For this review, take the finished solid that the model builds, in its own axes (mm). Face numbers are marked on the shaded views. Coordinates: 2 decimals unless noted, no trailing zeros. Write each loop counter-clockwise with the first axis right and the second up, starting at its lowest first coordinate (ties: lowest second). Pieces come first, ordered by that corner, then holes.
1) We need section A-A on x = 0. Write out the cut boundary in (y, z).
2) We need section C-C on y = 2.3. Write out the cut boundary in (x, z), then the cut area to 3 significant figures.
3) We need section D-D on y = 0.7. Write out the cut boundary in (x, z).
4) Insertion check: P1, Ø1.6, axis at y = 1.5, z = 3, coming from the -X side; P2, Ø1.5, axis at x = 7, z = -4.5, coming from the -Y side; P3, Ø1, axis at y = 2, z = -0.5, coming from the +X side. Each pin has a flat end and moves straight along its axis. Give the tip position at first contact, or say it passes through.
5) To check wall thickness, follow line 1 along X through (y, z) = (1.05, 0.25); line 2 along X through (y, z) = (1.8, -2.5); line 3 along Z through (x, y) = (-6, 1.55). State the ranges of each line that lie inside material, in increasing order.
6) We need section B-B on z = 0. Write out the cut boundary in (x, y).
7) Mouldability with a two-part tool opening along X and no side actions: class the marked faces 1 and 2 as pulls with the +X half, pulls with the -X half, needs draft (parallel to the pull), parting line crosses it, or undercut.
from build123d import *

# Parameters (mm, degrees)
SKETCH1_R             = 13
SKETCH1_W             = 15.2
SKETCH1_H             = 13
BOSS_EXTRUDE1_DEPTH   = 3
FILLET1_R             = 2
CHAMFER1_SIZE         = 1
CHAMFER1_SIZE2        = 0.577350269
CHAMFER1_PART_2_SIZE  = 1
CHAMFER1_PART_2_SIZE2 = 0.577350269
CHAMFER1_PART_3_SIZE  = 1
CHAMFER1_PART_3_SIZE2 = 0.577350269
CHAMFER1_PART_4_SIZE  = 1
CHAMFER1_PART_4_SIZE2 = 0.577350269


with BuildPart() as part:
    # Sketch1 → Boss-Extrude1 (new body)
    with BuildSketch(Plane(origin=(0, 0, 0), x_dir=(1, 0, 0), z_dir=(0, 1, 0))):
        Circle(SKETCH1_R)
        Rectangle(SKETCH1_W, SKETCH1_H, mode=Mode.SUBTRACT)
    extrude(amount=BOSS_EXTRUDE1_DEPTH)

    # Fillet1
    fillet1_edges = [part.edges().sort_by_distance(p)[0] for p in [
        (-13, 3, 0),
    ]]
    fillet(fillet1_edges, radius=FILLET1_R)

    # Chamfer1
    chamfer1_edges = [part.edges().sort_by_distance(p)[0] for p in [
        (-7.6, 0, 0),
    ]]
    chamfer1_side = [part.faces().sort_by_distance(p)[0] for p in [
        (-7.6, 1.5, 0),
    ]]
    chamfer(chamfer1_edges, length=CHAMFER1_SIZE, length2=CHAMFER1_SIZE2, reference=chamfer1_side[0])

    # Chamfer1 part 2
    chamfer1_part_2_edges = [part.edges().sort_by_distance(p)[0] for p in [
        (0, 0, 6.5),
    ]]
    chamfer1_part_2_side = [part.faces().sort_by_distance(p)[0] for p in [
        (0, 1.5, 6.5),
    ]]
    chamfer(chamfer1_part_2_edges, length=CHAMFER1_PART_2_SIZE, length2=CHAMFER1_PART_2_SIZE2, reference=chamfer1_part_2_side[0])

    # Chamfer1 part 3
    chamfer1_part_3_edges = [part.edges().sort_by_distance(p)[0] for p in [
        (7.6, 0, 0),
    ]]
    chamfer1_part_3_side = [part.faces().sort_by_distance(p)[0] for p in [
        (7.6, 1.5, 0),
    ]]
    chamfer(chamfer1_part_3_edges, length=CHAMFER1_PART_3_SIZE, length2=CHAMFER1_PART_3_SIZE2, reference=chamfer1_part_3_side[0])

    # Chamfer1 part 4
    chamfer1_part_4_edges = [part.edges().sort_by_distance(p)[0] for p in [
        (0, 0, -6.5),
    ]]
    chamfer1_part_4_side = [part.faces().sort_by_distance(p)[0] for p in [
        (0, 1.5, -6.5),
    ]]
    chamfer(chamfer1_part_4_edges, length=CHAMFER1_PART_4_SIZE, length2=CHAMFER1_PART_4_SIZE2, reference=chamfer1_part_4_side[0])


solid = part.part
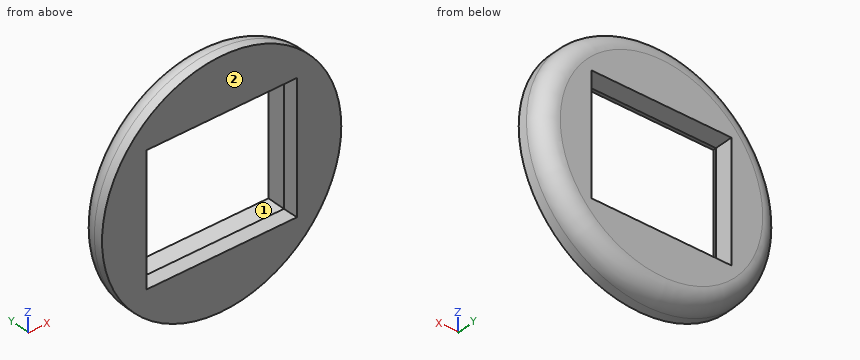
Result:
1. outline: (0, -13) - (1, -13) arc R2 ccw to (3, -11) - (3, -6.5) - (1, -6.5) - (0, -7.08) - close; (0, 7.08) - (1, 6.5) - (3, 6.5) - (3, 11) arc R2 ccw to (1, 13) - (0, 13) - close
2. outline: circle Ø25.04 at (0, 0); hole (-7.6, -6.5) - (7.6, -6.5) - (7.6, 6.5) - (-7.6, 6.5) - close
2. area: 295 mm2
3. outline: circle Ø26 at (0, 0); hole (-7.77, -6.67) - (7.77, -6.67) - (7.77, 6.67) - (-7.77, 6.67) - close
4. P1: stops at x = -12.79
4. P2: stops at y = 0.74
4. P3: stops at x = 12.93
5. line 1: x = -13 to -7.6, 7.6 to 13
5. line 2: x = -12.59 to -7.6, 7.6 to 12.59
5. line 3: z = -11.45 to -6.5, 6.5 to 11.45
6. outline: (-13, 0) - (-8.18, 0) - (-7.6, 1) - (-7.6, 3) - (-11, 3) arc R2 ccw to (-13, 1) - close; (7.6, 1) - (8.18, 0) - (13, 0) - (13, 1) arc R2 ccw to (11, 3) - (7.6, 3) - close
7. face 1: undercut
7. face 2: needs draft
